Could you check a few things on this model? Use its own coordinates, in mm. A direction names the side the tool comes from. Coordinates: 2 decimals unless noted, no trailing zeros. Loops run counter-clockwise (first coordinate to the right, second up) from the corner with the lowest first, then second, coordinate; pieces in that order, holes last. Notation, with made-up numbers: (85, -13.75) - (102, -13.75) arc R13 ccw to (102, -3.75) - close; hole circle Ø2 at (15.5, 20). An arc over 180 degrees is marked (long way). One line per item, written item: value. Start each with the question number.
(1) If we mould it in two halves opening along X, with no side actions, what happens to faces 1 (the face through (5.55, 2.57, 12.57)), 2 (the face through (-0.06, -6.07, 11.5)), 3 (the face through (-0.521, 1.966, -27.055))? For each: pulls with the +X half, pulls with the -X half, needs draft (parallel to the pull), parting line crosses it, or undercut.
(2) On a 3-axis mill with a long thin cutter (end or side, diameter ignored), from which of +Z, -Z, +X, -X, +Y, -Y can I reach the whole of each face in a straight line? I mean faces 4 (the face through (2, 0, 9)), 5 (the face through (0, 2, 13)), 6 (the face through (0, 3, -27)). Say none if no direction works.
(3) If I drill on line 1 along Y through (x, z) = (3, 4); line 2 along Y through (x, z) = (0, -26.25); line 3 along Z through (x, y) = (5, -4.25), over which ranges is the centre line in solid material (lowest first)? Write a range as from..to.
(4) If we section it at B-B on y = 0: Write out the boundary of the cut face in (x, z), then the cut area to 3 significant figures.
(5) If we section it at D-D on x = 2.5: Write out the boundary of the cut face in (y, z), then the cut area to 3 significant figures.
(6) I'm going to push flat-ended pins straight in: P1, Ø1.5, axis at y = -5, z = -26.5, coming from the +X side; P2, Ø9, axis at y = 0, z = 4, coming from the +X side; P3, Ø5, axis at x = -1, y = -5.5, coming from the -Z side. Where does each tip first touch, or does it pass through?
(7) If we section it at C-C on z = 4: Write out the boundary of the cut face in (x, y).
(8) If we section it at A-A on x = 0: Write out the boundary of the cut face in (y, z), then the cut area to 3 significant figures.
```python
from build123d import *

# Parameters (mm, degrees)
BOSS_EXTRUDE1_DEPTH = 6
SKETCH2_R           = 4
BOSS_EXTRUDE2_DEPTH = 40
CUT_EXTRUDE1_START  = -1
SKETCH3_R           = 5
CUT_EXTRUDE1_DEPTH  = 8
FILLET1_R           = 5
FILLET2_R           = 1.5


with BuildPart() as part:
    # Sketch1 → Boss-Extrude1 (new body, symmetric)
    with BuildSketch(Plane(origin=(0, 0, 0), x_dir=(0, 0, -1), z_dir=(1, 0, 0))):
        Polygon((13, 7.5), (17, -7.5), (-13, -7.5), (-13, 7.5), align=None)
    extrude(amount=BOSS_EXTRUDE1_DEPTH, both=True)

    # Sketch2 → Boss-Extrude2 (add)
    with BuildSketch(Plane.XY):
        with BuildLine():
            Line((-1, -7.5), (1, -7.5))
            Line((1, -7.5), (1, -6.898979486))
            ThreePointArc((1, -6.898979486), (0, 3), (-1, -6.898979486))
            Line((-1, -6.898979486), (-1, -7.5))
        make_face()
        with Locations((0, -2)):
            Circle(SKETCH2_R, mode=Mode.SUBTRACT)
    extrude(amount=-BOSS_EXTRUDE2_DEPTH)

    # Sketch3 → Cut-Extrude1 (cut, through all)
    with BuildSketch(Plane(origin=(0, 0, 0), x_dir=(0, 0, -1), z_dir=(1, 0, 0)).offset(CUT_EXTRUDE1_START)):
        with Locations((-4, 0)):
            Circle(SKETCH3_R)
    extrude(amount=CUT_EXTRUDE1_DEPTH, mode=Mode.SUBTRACT)

    # Fillet1
    fillet1_edges = [part.edges().sort_by_distance(p)[0] for p in [
        (0, -7.5, 13),
    ]]
    fillet(fillet1_edges, radius=FILLET1_R)

    # Fillet2
    fillet2_edges = [part.edges().sort_by_distance(p)[0] for p in [
        (6, -7.5, -4.5),
        (-6, -7.5, -4.5),
        (-6, -6.035533906, 11.535533906),
        (6, -6.035533906, 11.535533906),
        (6, 7.5, 0),
        (-6, 2.5, 13),
        (-6, 7.5, 0),
        (6, 2.5, 13),
    ]]
    fillet(fillet2_edges, radius=FILLET2_R)


solid = part.part
```
Values:
1. face 1: pulls with the +X half
1. face 2: needs draft
1. face 3: undercut
2. face 4: +X
2. face 5: +Z, +X, -X, +Y, -Y
2. face 6: -Z
3. line 1: y = -7.5..-5, 5..7.5
3. line 2: y = -7.5..-6, 2..3
3. line 3: z = -16.13..1.37, 6.63..12.59
4. outline: (-6, -15) - (-4.58, -15) - (-4.58, -40) - (-3.46, -40) - (-3.46, -15) - (3.46, -15) - (3.46, -40) - (4.58, -40) - (4.58, -15) - (6, -15) - (6, -1) - (-1, -1) - (-1, 9) - (6, 9) - (6, 11.5) arc R1.5 ccw to (4.5, 13) - (-4.5, 13) arc R1.5 ccw to (-6, 11.5) - close
4. area: 321 mm2
5. outline: (-7.5, -17) - (-6.33, -16.69) - (-6.33, -40) - (-5.12, -40) - (-5.12, -16.37) - (1.12, -14.7) - (1.12, -40) - (2.33, -40) - (2.33, -14.38) - (7.5, -13) - (7.5, 13) - (-2.5, 13) arc R5 ccw to (-7.5, 8) - close; hole circle Ø10 at (0, 4)
5. area: 395 mm2
6. P1: stops at x = 4.47
6. P2: stops at x = -1
6. P3: stops at z = -40
7. outline: (-6, -6) arc R1.5 ccw to (-4.5, -7.5) - (4.5, -7.5) arc R1.5 ccw to (6, -6) - (6, -5) - (-1, -5) - (-1, 5) - (6, 5) - (6, 6) arc R1.5 ccw to (4.5, 7.5) - (-4.5, 7.5) arc R1.5 ccw to (-6, 6) - close
8. outline: (-7.5, -40) - (-6, -40) - (-6, -16.6) - (2, -14.47) - (2, -40) - (3, -40) - (3, -14.2) - (7.5, -13) - (7.5, 13) - (-2.5, 13) arc R5 ccw to (-7.5, 8) - close; hole circle Ø10 at (0, 4)
8. area: 397 mm2
